Build history of the part. All positions in model axes, mm. Face numbers are marked on the shaded views. A direction names the side the tool comes from. Give positions to 0.01 mm unless a question says otherwise; leave off trailing zeros. Write each loop counter-clockwise with the first axis right and the second up, starting at its lowest first coordinate (ties: lowest second). Pieces come first, ordered by that corner, then holes. Notation, with made-up numbers: (78, 33) -> (94, 33) arc R14 cw to (94, 48) -> close; hole circle Ø2 at (25.5, 87.5). An arc over 180 degrees is marked (long way). Put each result on its own line as item: value. Start each with the question number.
Item 1: Two-plate mould, pull along Y, no slides. Class the marked faces 1, 2 and 3: pulls with the +Y half, pulls with the -Y half, needs draft (parallel to the pull), parting line crosses it, or undercut.
Item 2: Slice it at B-B, the plane y = 352. List the corners of the cut face in (x, z).
Item 3: Drill centre lines: line 1 along X through (y, z) = (414, 118); line 2 along X through (y, z) = (296.5, 81); line 3 along Y through (x, z) = (289, 111). Where is each one in solid material? Low to high.
Item 4: Slice it at C-C, the plane x = 1054.5. List the corners of the cut face in (y, z), plus the area to 3 significant figures.
Item 5: Tool access for the marked faces 4 and 5: list every direction of +Z, -Z, +X, -X, +Y, -Y with a clear straight run to the whole face (end or side of a thin tool).
Item 6: Slice it at A-A, the plane z = 107. List the corners of the cut face in (x, y), plus the area to 4 significant figures.
Item 7: Slice it at D-D, the plane y = 424. List the corners of the cut face in (x, z), plus the area to 3 significant figures.
Item 8: Flat gauge pin, fed straight in: pin 1 Ø5 at (x, y) = (1068, 228) entering from +Z. Where does the tip first touch, or does it go through?
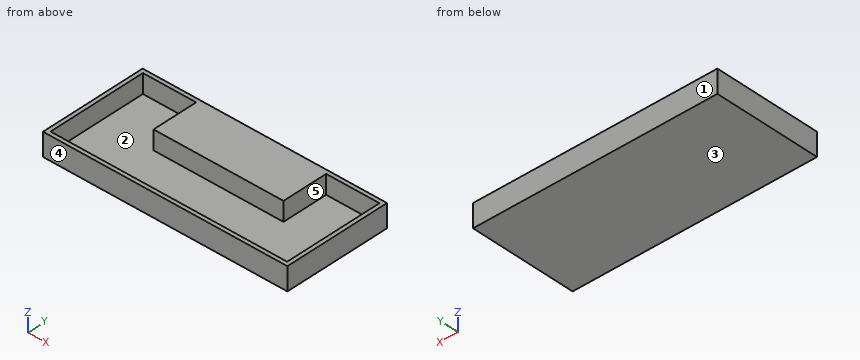
```python
from build123d import *

# Parameters (mm, degrees)
F1_DEPTH = 150
F3_T     = -25.4
F2_W     = 800
F2_H     = 300
F4_DEPTH = 150


with BuildPart() as f1:
    # F0 (on Top) → F1 (new body)
    with BuildSketch(Plane.XY):
        Polygon((0, 700), (0, 0), (1600, 0), (1600, 700), (1200, 700), (1200, 400), (400, 400), (400, 700), align=None)
    extrude(amount=F1_DEPTH)

    # F3
    f3_openings = [f1.faces().sort_by_distance(p)[0] for p in [
        (800, 295.454545, 150),
    ]]
    offset(amount=F3_T, openings=f3_openings, kind=Kind.INTERSECTION)

    # F2 (on Top) → F4 (join)
    with BuildSketch(Plane.XY):
        with Locations((800, 550)):
            Rectangle(F2_W, F2_H)
    extrude(amount=F4_DEPTH)


solid = f1.part
```
Values follow:
1. face 1: pulls with the +Y half
1. face 2: undercut
1. face 3: needs draft
2. outline: (0, 0) -> (1600, 0) -> (1600, 150) -> (1574.6, 150) -> (1574.6, 25.4) -> (25.4, 25.4) -> (25.4, 150) -> (0, 150) -> close
3. line 1: 0 to 25.4, 374.6 to 1225.4, 1574.6 to 1600
3. line 2: 0 to 25.4, 1574.6 to 1600
3. line 3: 0 to 25.4, 674.6 to 700
4. outline: (0, 0) -> (700, 0) -> (700, 150) -> (374.6, 150) -> (374.6, 25.4) -> (25.4, 25.4) -> (25.4, 150) -> (0, 150) -> close
4. area: 61,500 mm2
5. face 4: +Z, -Z, +X, -X, -Y
5. face 5: +Z
6. outline: (0, 0) -> (1600, 0) -> (1600, 700) -> (0, 700) -> close; hole (25.4, 25.4) -> (1574.6, 25.4) -> (1574.6, 674.6) -> (1225.4, 674.6) -> (1225.4, 374.6) -> (374.6, 374.6) -> (374.6, 674.6) -> (25.4, 674.6) -> close
6. area: 369,500 mm2
7. outline: (0, 0) -> (1600, 0) -> (1600, 150) -> (1574.6, 150) -> (1574.6, 25.4) -> (1225.4, 25.4) -> (1225.4, 150) -> (374.6, 150) -> (374.6, 25.4) -> (25.4, 25.4) -> (25.4, 150) -> (0, 150) -> close
7. area: 153,000 mm2
8. pin 1: z = 25.4
